Source: CAD feature listing. Evaluate the final solid. Frame: model axes, mm. Coordinates: 2 decimals unless noted, no trailing zeros. Order: outer loops, then holes, each group sorted by start corner. A loop starts at its lowest first (then second) coordinate and runs counter-clockwise, first axis right, second up.
Item 1: Mould query, pull axis X, two halves, no side actions, for faces 1 (the flat face through (0, -2, 0)), 2 (the cylindrical face through (10, 3.2, 15.3)), 3 (the cylindrical face through (0.133, 1.016, 15.283)). Classes: released by +X, released by -X, zero draft, split by the parting line, or undercut.
Item 2: Contact query for flat-ended pins moving along their axis: P1, Ø4, axis at x = -5, z = 14.5, coming from the -Y side; P2, Ø5, axis at y = 6.5, z = 7, coming from the -X side; P3, Ø1.5, axis at x = -6.5, z = 8.5, coming from the +Y side. Output: stop coordinate, or through.
Item 3: Section C-C on z = 15. Return the cut outline in (x, y) (3 decimals), then the cut area to 3 significant figures.
Item 4: Ray query, line 1 (Y direction, x = 0, z = 20) (3 decimals); line 2 (Y direction, x = 5.5, z = 24); line 3 (X direction, y = 5, z = 10.5). Return the intervals inside material, ascending.
Item 5: Section A-A on y = 0. Return the cut outline in (x, z) (3 decimals).
from build123d import *

# Parameters (mm, degrees)
SKETCH1_R           = 10.5
BOSS_EXTRUDE1_DEPTH = 31
FILLET1_R           = 1.5
SKETCH2_R           = 1.025
CUT_EXTRUDE1_DEPTH  = 35


with BuildPart() as part:
    # Sketch1 → Boss-Extrude1 (new body)
    with BuildSketch(Plane.XY):
        Circle(SKETCH1_R)
    extrude(amount=BOSS_EXTRUDE1_DEPTH)

    # Fillet1
    fillet1_edges = [part.edges().sort_by_distance(p)[0] for p in [
        (-10.5, 0, 0),
        (-10.5, 0, 31),
    ]]
    fillet(fillet1_edges, radius=FILLET1_R)

    # Sketch2 → Cut-Extrude1 (cut)
    with BuildSketch(Plane(origin=(0, 0, 0), x_dir=(-1, 0, 0), z_dir=(0, 0, -1))):
        Circle(SKETCH2_R)
    extrude(amount=-CUT_EXTRUDE1_DEPTH, mode=Mode.SUBTRACT)


solid = part.part
Answer list:
1. face 1: zero draft
1. face 2: split by the parting line
1. face 3: undercut
2. P1: stops at y = -10.06
2. P2: stops at x = -9.71
2. P3: stops at y = 8.79
3. outline: circle Ø21 at (0, 0); hole circle Ø2.05 at (0, 0)
3. area: 343 mm2
4. line 1: y = -10.5 to -1.025, 1.025 to 10.5
4. line 2: y = -8.94 to 8.94
4. line 3: x = -9.23 to 9.23
5. outline: (-10.5, 1.5) arc R1.5 ccw to (-9, 0) - (-1.025, 0) - (-1.025, 31) - (-9, 31) arc R1.5 ccw to (-10.5, 29.5) - close; (1.025, 0) - (9, 0) arc R1.5 ccw to (10.5, 1.5) - (10.5, 29.5) arc R1.5 ccw to (9, 31) - (1.025, 31) - close
